Work out the finished part from the listing and answer in its coordinate system (mm). A direction names the side the tool comes from. Round coordinates to 2 decimals unless told otherwise and drop trailing zeros. Loops run counter-clockwise (first coordinate to the right, second up) from the corner with the lowest first, then second, coordinate; pieces in that order, holes last. Notation, with made-up numbers: (58, 16.25) - (93, 16.25) arc R9 cw to (93, 33.25) - close; hole circle Ø8 at (-35, 72.5). An arc over 180 degrees is marked (long way). Return JSON: item names as keys, results as strings.
from build123d import *

# Parameters (mm, degrees)
SKETCH1_W               = 207.01
SKETCH1_H               = 171.45
BOSS_EXTRUDE1_DEPTH     = 69.85
CUT_EXTRUDE1_DEPTH      = 68.58
CUT_EXTRUDE2_DEPTH      = 1
CUT_EXTRUDE2_DEPTH_BACK = 70.85
FILLET3_R               = 2.54


with BuildPart() as part:
    # Sketch1 → Boss-Extrude1 (new body)
    with BuildSketch(Plane(origin=(0, 0, 0), x_dir=(1, 0, 0), z_dir=(0, 1, 0))):
        with Locations((103.505, -85.725)):
            Rectangle(SKETCH1_W, SKETCH1_H)
    extrude(amount=BOSS_EXTRUDE1_DEPTH)

    # Sketch3 → Cut-Extrude1 (cut)
    with BuildSketch(Plane(origin=(0, 69.85, 0), x_dir=(1, 0, 0), z_dir=(0, 1, 0))):
        Polygon((1.905, -93.98), (41.499681461, -71.12), (1.905, -71.12), align=None)
        Polygon((41.91, -76.230101608), (1.905, -99.326999127), (1.905, -145.520794165), (41.91, -168.617691684), (81.915, -145.520794165), (81.915, -99.326999127), (71.846181898, -93.513764285), (73.116181898, -91.314059759), (81.915, -96.394059759), (90.713818102, -91.314059759), (91.983818102, -93.513764285), (84.455, -97.860529443), (84.455, -144.054324481), (124.46, -167.151222), (164.465, -144.054324481), (164.465, -97.860529443), (124.46, -74.763631924), (114.391181898, -80.576866766), (113.121181898, -78.377162241), (121.92, -73.297162241), (121.92, -63.137162241), (124.46, -63.137162241), (124.46, -71.830692557), (164.465, -94.927590076), (204.47, -71.830692557), (204.47, -25.636897519), (164.465, -2.54), (124.46, -25.636897519), (124.46, -37.263367203), (121.92, -37.263367203), (121.92, -27.103367203), (81.915, -4.006469684), (41.91, -27.103367203), (41.91, -37.263367203), (35.56, -37.263367203), (35.56, -6.35), (5.08, -6.35), (5.08, -41.91), (35.56, -41.91), (35.56, -46.99), (13.97, -46.99), (13.97, -68.58), (35.56, -68.58), (35.56, -63.137162241), (41.91, -63.137162241), (41.91, -73.297162241), (50.708818102, -78.377162241), (49.438818102, -80.576866766), align=None)
        Polygon((37.465, -24.765), (75.959829198, -2.54), (37.465, -2.54), align=None)
        Polygon((167.075023065, -2.54), (204.47, -24.13), (204.47, -2.54), align=None)
        Polygon((82.645969059, -2.54), (121.92, -24.592453018), (160.115969059, -2.54), align=None)
    extrude(amount=-CUT_EXTRUDE1_DEPTH, mode=Mode.SUBTRACT)

    # Sketch4 → Cut-Extrude2 (cut, two sides)
    with BuildSketch(Plane(origin=(0, 69.85, 0), x_dir=(1, 0, 0), z_dir=(0, 1, 0))) as cut_extrude2_sk:
        Polygon((207.01, -74.315776706), (167.005, -97.412674225), (167.005, -146.601672765), (123.966434747, -171.45), (167.005, -171.45), (207.01, -171.45), align=None)
        Polygon((0, -147.53821025), (41.416434747, -171.45), (0, -171.45), align=None)
        Polygon((41.670434747, -171.45), (123.712434747, -171.45), (82.691434747, -147.766514608), align=None)
        Polygon((81.915, -9.872348419), (46.99, -30.03630657), (46.99, -70.364222873), (81.915, -90.528181024), (116.84, -70.364222873), (116.84, -30.03630657), align=None)
        Polygon((164.465, -8.405878735), (129.54, -28.569836886), (129.54, -68.897753189), (164.465, -89.061711341), (199.39, -68.897753189), (199.39, -28.569836886), align=None)
        Polygon((41.91, -82.095980343), (6.985, -102.259938494), (6.985, -142.587854797), (41.91, -162.751812949), (76.835, -142.587854797), (76.835, -102.259938494), align=None)
        Polygon((124.46, -80.629510659), (89.535, -100.793468811), (89.535, -141.121385114), (124.46, -161.285343265), (159.385, -141.121385114), (159.385, -100.793468811), align=None)
    extrude(amount=CUT_EXTRUDE2_DEPTH, mode=Mode.SUBTRACT)
    extrude(cut_extrude2_sk.sketch, amount=-CUT_EXTRUDE2_DEPTH_BACK, mode=Mode.SUBTRACT)

    # Fillet3
    fillet3_edges = [part.edges().sort_by_distance(p)[0] for p in [
        (0, 34.925, 147.53821025),
        (82.691434747, 34.925, 147.766514608),
        (207.01, 34.925, 74.315776706),
        (167.005, 34.925, 146.601672765),
        (167.005, 34.925, 97.412674225),
        (0, 34.925, 0),
        (207.01, 34.925, 0),
    ]]
    fillet(fillet3_edges, radius=FILLET3_R)


solid = part.part
1) Find the intervals of material crossed by L1, parallel to X at y = 12, z = 132.5 (3 decimals); L2, parallel to X at y = 58.5, z = 34.5; L3, parallel to Z at x = 96, y = 6, in increasing order.
Verdict:
{"L1": "x = 0 to 1.905, 81.915 to 84.455, 164.465 to 167.005", "L2": "x = 0 to 5.08, 35.56 to 41.91, 121.92 to 124.46, 204.47 to 207.01", "L3": "z = 0 to 2.54, 10.04 to 12.14, 150.72 to 155.45"}
2) Section D-D (z = 52.5) is taken. Give the vertices of the cut face in (x, y), and give its area (3 significant figures).
Verdict:
{"outline": "(0, 0) - (46.99, 0) - (46.99, 1.27) - (13.97, 1.27) - (13.97, 69.85) - (0, 69.85) - close; (116.84, 0) - (129.54, 0) - (129.54, 1.27) - (116.84, 1.27) - close; (199.39, 0) - (207.01, 0) - (207.01, 69.85) - (204.47, 69.85) - (204.47, 1.27) - (199.39, 1.27) - close", "area": "1,220 mm2"}
3) Section C-C (x = 174) is taken. Give the vertices of the cut face in (y, z), and give its area (3 significant figures).
Verdict:
{"outline": "(0, 0) - (69.85, 0) - (69.85, 2.54) - (1.27, 2.54) - (1.27, 6.54) - (69.85, 6.54) - (69.85, 8.05) - (1.27, 8.05) - (1.27, 13.91) - (0, 13.91) - close; (0, 83.56) - (1.27, 83.56) - (1.27, 89.42) - (69.85, 89.42) - (69.85, 93.37) - (0, 93.37) - close", "area": "579 mm2"}
4) Section A-A (z = 104.5) is taken. Give the vertices of the cut face in (x, y) (3 decimals).
Verdict:
{"outline": "(0, 0) - (6.985, 0) - (6.985, 1.27) - (1.905, 1.27) - (1.905, 69.85) - (0, 69.85) - close; (76.835, 0) - (89.535, 0) - (89.535, 1.27) - (84.455, 1.27) - (84.455, 69.85) - (81.915, 69.85) - (81.915, 1.27) - (76.835, 1.27) - close; (159.385, 0) - (167.005, 0) - (167.005, 69.85) - (164.465, 69.85) - (164.465, 1.27) - (159.385, 1.27) - close"}
5) A tool of negligible diameter and unlimited length cuts with its end or side. For faces 1 (the flat face through (187.27, 35.414, 85.713)), 2 (the flat face through (146.76, 0.64, 78.84)), 3 (the flat face through (61.824, 35.414, 159.814)), 4 (the flat face through (121.92, 36, 68)), 5 (the flat face through (0, 34, 75)), from which of +Z, -Z, +X, -X, +Y, -Y can it reach the whole face along a straight path? Write none if from no direction.
Verdict:
{"face 1": "+Z, +X, +Y, -Y", "face 2": "+Y, -Y", "face 3": "+Z, +Y, -Y", "face 4": "+Y", "face 5": "+Z, -Z, -X, +Y, -Y"}
6) Section B-B (x = 96.5) is taken. Give the vertices of the cut face in (y, z), and give its area (3 significant figures).
Verdict:
{"outline": "(0, 0) - (69.85, 0) - (69.85, 2.54) - (1.27, 2.54) - (1.27, 10.32) - (69.85, 10.32) - (69.85, 12.43) - (1.27, 12.43) - (1.27, 18.29) - (0, 18.29) - close; (0, 82.11) - (1.27, 82.11) - (1.27, 96.77) - (0, 96.77) - close; (0, 145.14) - (1.27, 145.14) - (1.27, 151.01) - (69.85, 151.01) - (69.85, 155.74) - (0, 155.74) - close", "area": "698 mm2"}
7) Flat-ended cylindrical pins translate along their axes: pin 1 (8 mm diameter, centred on y = 41.5, z = 148, fed in from -X); pin 2 (0.8 mm diameter, centred on x = 123, y = 47, fed in from +Z); pin 3 (3 mm diameter, centred on x = 56, z = 91.5, fed in from +Y); pin 4 (11.5 mm diameter, centred on x = 50, y = 37.5, fed in from +Z). Find the tip coordinate at first contact, or state that the pin passes through.
Verdict:
{"pin 1": "stops at x = 0", "pin 2": "stops at z = 171.27", "pin 3": "stops at y = 1.27", "pin 4": "stops at z = 169.96"}
